from build123d import *

# Parameters (mm, degrees)
SKETCH_1_R      = 1.6
EXTRUDE_1_DEPTH = 3
SKETCH_3_W      = 15.866394843
SKETCH_3_H      = 55.981711963
SKETCH_3_W_2    = 12.02170443
SKETCH_3_H_2    = 38.866282165
EXTRUDE_3_DEPTH = 3


with BuildPart() as part:
    # 草图1 → 凸台-拉伸1 (new body)
    with BuildSketch(Plane(origin=(0, 0, 0), x_dir=(1, 0, 0), z_dir=(0, 1, 0))):
        with BuildLine():
            Line((-80.009028181, 21.402670377), (-80.009028181, -28.604431477))
            ThreePointArc((-80.009028181, -28.604431477), (-79.134066788, -30.716775138), (-77.021723127, -31.591736531))
            Line((-77.021723127, -31.591736531), (12.787258331, -31.591736531))
            ThreePointArc((12.787258331, -31.591736531), (14.899601993, -30.716775138), (15.774563386, -28.604431477))
            Line((15.774563386, -28.604431477), (15.774563386, 21.402670377))
            ThreePointArc((15.774563386, 21.402670377), (14.899601993, 23.515014039), (12.787258331, 24.389975432))
            Line((12.787258331, 24.389975432), (-77.021723127, 24.389975432))
            ThreePointArc((-77.021723127, 24.389975432), (-79.134066788, 23.515014039), (-80.009028181, 21.402670377))
        make_face()
        with Locations(Location((-76.52848462, 20.886724226, 0), (0, 0, 270))):
            Circle(SKETCH_1_R, mode=Mode.SUBTRACT)
        with Locations(Location((-18.52858622, 20.886597225, 0), (0, 0, 270))):
            Circle(SKETCH_1_R, mode=Mode.SUBTRACT)
        with Locations(Location((-18.52833222, -28.113656775, 0), (0, 0, 270))):
            Circle(SKETCH_1_R, mode=Mode.SUBTRACT)
        with Locations(Location((-76.52833222, -28.113529775, 0), (0, 0, 270))):
            Circle(SKETCH_1_R, mode=Mode.SUBTRACT)
        with BuildLine():
            Line((-70.903401709, 18.230282987), (-54.564490165, 18.082300473))
            ThreePointArc((-54.564490165, 18.082300473), (-53.860065027, 17.78301522), (-53.573587867, 17.073284796))
            Line((-53.573587867, 17.073284796), (-53.940568984, -23.445502526))
            ThreePointArc((-53.940568984, -23.445502526), (-54.239854236, -24.149927664), (-54.94958466, -24.436404824))
            Line((-54.94958466, -24.436404824), (-71.288496204, -24.288422311))
            ThreePointArc((-71.288496204, -24.288422311), (-71.992921342, -23.989137058), (-72.279398502, -23.279406634))
            Line((-72.279398502, -23.279406634), (-71.912417386, 17.239380688))
            ThreePointArc((-71.912417386, 17.239380688), (-71.613132133, 17.943805826), (-70.903401709, 18.230282987))
        make_face(mode=Mode.SUBTRACT)
    extrude(amount=EXTRUDE_1_DEPTH)

    # 草图3 → 凸台-拉伸3 (add)
    with BuildSketch(Plane.XZ):
        with Locations((-7.293882236, 3.60088055)):
            Rectangle(SKETCH_3_W, SKETCH_3_H)
        with Locations((-30.854956036, 3.919082923)):
            Rectangle(SKETCH_3_W_2, SKETCH_3_H_2)
    extrude(amount=EXTRUDE_3_DEPTH)


solid = part.part
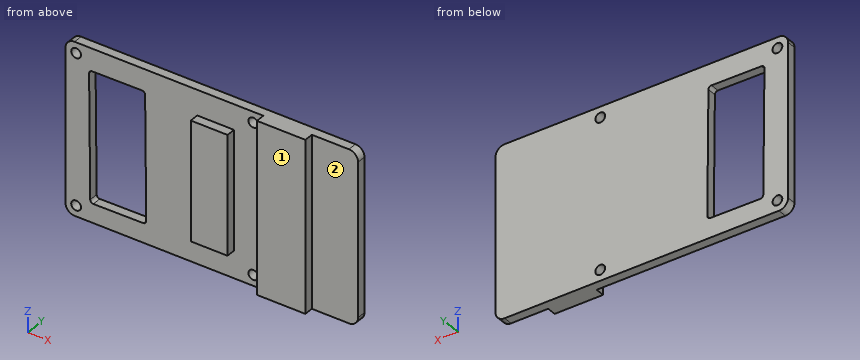
Part model, mm, in its own coordinate system. Face numbers are marked on the shaded views. A direction names the side the tool comes from. Coordinates: 2 decimals unless noted, no trailing zeros. Loops run counter-clockwise (first coordinate to the right, second up) from the corner with the lowest first, then second, coordinate; pieces in that order, holes last. Notation, with made-up numbers: M -15.5,2.5 L 30.5,2.5 A36 cw 30.5,39.5 Z; hole C -30.75,18 d7. An arc over 180 degrees is marked long. Use a Markdown table: item, result. Add a question column.
Q1. Cut at D-D (x = -35). Write the cut outline in (y, z), and give its area (3 significant figures).
Q2. Probe L1, parallel to X at y = -0.2, z = 11.5; L2, parallel to X at y = 0.7, z = 21.5; L3, parallel to X at y = -1, z = -21. List the from-to ranges inside material, lowest first.
Q3. Which spindle directions (+Z, -Z, +X, -X, +Y, -Y) get a long thin tool onto all of the face, cutting with end or side? Do the marked faces 1 and 2. Say none if no direction does.
Q4. Pin check, flat tips, straight feed: P1, Ø7.5, axis at x = 8, z = 5.5, coming from the -Y side; P2, Ø3.5, axis at y = -2, z = 9.5, coming from the +X side; P3, Ø3.5, axis at y = -2, z = 8.5, coming from the -X side. Stop position of each tip, or through.
Q5. Cut at B-B (x = -61.5). Write the cut outline in (y, z).
Q6. Cut at A-A (y = -2). Write the cut outline in (x, z), and give its area (3 significant figures).
Q7. Cut at C-C (z = 14). Write the cut outline in (x, y), and give its area (3 significant figures).
Worked out:
| question | item | result |
|---|---|---|
| 1 | outline | M -3,-15.51 L 0,-15.51 L 0,-24.39 L 3,-24.39 L 3,31.59 L 0,31.59 L 0,23.35 L -3,23.35 Z |
| 1 | area | 285 mm2 |
| 2 | L1 | x = -36.87 to -24.84, -15.23 to 0.64 |
| 2 | L2 | x = -80.01 to -72.26, -53.92 to 15.77 |
| 2 | L3 | x = -15.23 to 0.64 |
| 3 | face 1 | +Z, -Z, +X, -X, -Y |
| 3 | face 2 | +Z, -Z, +X, -Y |
| 4 | P1 | stops at y = 0 |
| 4 | P2 | stops at x = 0.64 |
| 4 | P3 | stops at x = -36.87 |
| 5 | outline | M 0,-24.39 L 3,-24.39 L 3,-18.15 L 0,-18.15 Z; M 0,24.38 L 3,24.38 L 3,31.59 L 0,31.59 Z |
| 6 | outline | M -36.87,-15.51 L -24.84,-15.51 L -24.84,23.35 L -36.87,23.35 Z; M -15.23,-24.39 L 0.64,-24.39 L 0.64,31.59 L -15.23,31.59 Z |
| 6 | area | 1,360 mm2 |
| 7 | outline | M -80.01,0 L -72.2,0 L -72.2,3 L -80.01,3 Z; M -53.86,0 L -36.87,0 L -36.87,-3 L -24.84,-3 L -24.84,0 L -15.23,0 L -15.23,-3 L 0.64,-3 L 0.64,0 L 15.77,0 L 15.77,3 L -53.86,3 Z |
| 7 | area | 316 mm2 |
